For this review, take the finished solid that the model builds, in its own axes (mm). Face numbers are marked on the shaded views. A direction names the side the tool comes from. Give positions to 0.01 mm unless a question says otherwise; leave off trailing zeros. Order: outer loops, then holes, each group sorted by start corner. A loop starts at its lowest first (then second) coordinate and runs counter-clockwise, first axis right, second up.
Item 1: Consider section A-A (y = 9.5). Give the boundary of the cut face in (x, z), plus the area to 3 significant figures.
Item 2: Consider section B-B (z = 10). Give the boundary of the cut face in (x, y).
Item 3: Consider section D-D (z = 14.25). Give the boundary of the cut face in (x, y), plus the area to 3 significant figures.
Item 4: Machinability: for the marked faces 1, 2, 3, 4 and 5, which of the approach directions +Z, -Z, +X, -X, +Y, -Y give a long, thin tool a straight path to every point of the face, cutting with its end or side? Answer none if there is none.
Item 5: For probe 1 along Z at (x, y) = (-21, -12.75); probe 2 along X at (y, z) = (-0.25, 14); probe 3 along Z at (x, y) = (-2, 10), list the stretches that pass through material, from the lowest coordinate up.
Item 6: The part is to be moulded in two halves that separate along X. For the marked faces 6, 7 and 8, say which applies: released by +X, released by -X, zero draft, split by the parting line, or undercut.
Item 7: Consider section C-C (x = 0). Give the boundary of the cut face in (y, z).
Item 8: For P1, Ø6, axis at y = 5.5, z = 10, coming from the +X side; P2, Ø8, axis at y = 9, z = 9.5, coming from the -X side; P3, Ø3, axis at x = -19.5, z = 6, coming from the +Y side, all flat-tipped, find the tip position at first contact; note any pin that passes through.
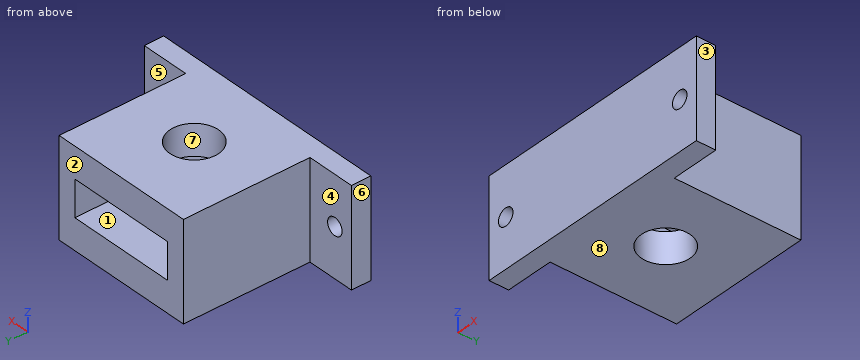
```python
from build123d import *

# Parameters (mm, degrees)
SKETCH2_W           = 30
SKETCH2_H           = 30
SKETCH2_R           = 5
BOSS_EXTRUDE1_DEPTH = 20
CUT_EXTRUDE2_START  = 10
CUT_EXTRUDE2_DEPTH  = 3.7
SKETCH4_W           = 10
SKETCH4_H           = 20
SKETCH4_R           = 1.75
BOSS_EXTRUDE2_DEPTH = 4


with BuildPart() as part:
    # Sketch2 → Boss-Extrude1 (new body)
    with BuildSketch(Plane.XY):
        Rectangle(SKETCH2_W, SKETCH2_H)
        Circle(SKETCH2_R, mode=Mode.SUBTRACT)
    extrude(amount=BOSS_EXTRUDE1_DEPTH)

    # Sketch3 → Cut-Extrude2 (cut, symmetric)
    with BuildSketch(Plane.XY.offset(CUT_EXTRUDE2_START)):
        with BuildLine():
            Line((-11.2, 15), (-11.2, 0))
            ThreePointArc((-11.2, 0), (0, -11.2), (11.2, 0))
            Line((11.2, 0), (11.2, 15))
            Line((11.2, 15), (-11.2, 15))
        make_face()
    extrude(amount=CUT_EXTRUDE2_DEPTH, both=True, mode=Mode.SUBTRACT)

    # Sketch4 → Boss-Extrude2 (add)
    with BuildSketch(Plane.XZ.offset(15)):
        with Locations((-20, 10)):
            Rectangle(SKETCH4_W, SKETCH4_H)
        with Locations((-21, 10)):
            Circle(SKETCH4_R, mode=Mode.SUBTRACT)
        with Locations((20, 10)):
            Rectangle(SKETCH4_W, SKETCH4_H)
        with Locations((21, 10)):
            Circle(SKETCH4_R, mode=Mode.SUBTRACT)
    extrude(amount=-BOSS_EXTRUDE2_DEPTH)


solid = part.part
```
Resolved:
1. outline: (-15, 0) - (15, 0) - (15, 20) - (-15, 20) - close; hole (-11.2, 6.3) - (11.2, 6.3) - (11.2, 13.7) - (-11.2, 13.7) - close
1. area: 434 mm2
2. outline: (-25, -15) - (-22.75, -15) - (-22.75, -11) - (-25, -11) - close; (-19.25, -15) - (19.25, -15) - (19.25, -11) - (15, -11) - (15, 15) - (11.2, 15) - (11.2, 0) arc R11.2 cw to (-11.2, 0) - (-11.2, 15) - (-15, 15) - (-15, -11) - (-19.25, -11) - close; (22.75, -15) - (25, -15) - (25, -11) - (22.75, -11) - close
3. outline: (-25, -15) - (25, -15) - (25, -11) - (15, -11) - (15, 15) - (-15, 15) - (-15, -11) - (-25, -11) - close; hole circle Ø10 at (0, 0)
3. area: 901 mm2
4. face 1: +Y
4. face 2: +Z, -Z, +X, -X, +Y
4. face 3: +Z, -Z, +X, +Y, -Y
4. face 4: +Z, -Z, -X, +Y
4. face 5: +Z, -Z, +X, +Y
5. probe 1: z = 0 to 8.25, 11.75 to 20
5. probe 2: x = -15 to -4.99, 4.99 to 15
5. probe 3: z = 0 to 6.3, 13.7 to 20
6. face 6: released by -X
6. face 7: undercut
6. face 8: zero draft
7. outline: (-15, 0) - (-5, 0) - (-5, 6.3) - (-11.2, 6.3) - (-11.2, 13.7) - (-5, 13.7) - (-5, 20) - (-15, 20) - close; (5, 0) - (15, 0) - (15, 6.3) - (5, 6.3) - close; (5, 13.7) - (15, 13.7) - (15, 20) - (5, 20) - close
8. P1: stops at x = 15
8. P2: stops at x = -15
8. P3: stops at y = -11
